The model under review builds one solid part; all positions refer to its coordinate system, in mm. A direction names the side the tool comes from. Round coordinates to 2 decimals unless told otherwise and drop trailing zeros. Loops run counter-clockwise (first coordinate to the right, second up) from the corner with the lowest first, then second, coordinate; pieces in that order, holes last. Notation, with made-up numbers: M -30,38 L -11,38 A24 ccw -11,65 Z; hole C 62.5,38.25 d4. An arc over 180 degrees is marked long. Answer in a Markdown table with one row per item. Add a question column.
from build123d import *

# Parameters (mm, degrees)
SKETCH2_W             = 31.8
SKETCH2_H             = 15.8
SKETCH2_W_2           = 29.4
SKETCH2_H_2           = 13.4
BOSS_EXTRUDE1_DEPTH   = 3.2
SKETCH2_3_R           = 3.255
SKETCH2_3_R_2         = 2.4
BOSS_EXTRUDE2_DEPTH   = 2.2
BOSS_EXTRUDE2_2_DEPTH = 2.2
BOSS_EXTRUDE2_3_DEPTH = 2.2
SKETCH3_W             = 29.4
SKETCH3_H             = 13.4
BOSS_EXTRUDE3_DEPTH   = 1
SKETCH4_R             = 2.4
SKETCH4_R_2           = 2.399999999
BOSS_EXTRUDE4_DEPTH   = 1.8
SKETCH5_R             = 1.3
CUT_EXTRUDE1_DEPTH    = 1.8


with BuildPart() as part:
    # Sketch2 → Boss-Extrude1 (new body)
    with BuildSketch(Plane.XY):
        with Locations((15.9, -7.9)):
            Rectangle(SKETCH2_W, SKETCH2_H)
        with Locations((15.9, -7.9)):
            Rectangle(SKETCH2_W_2, SKETCH2_H_2, mode=Mode.SUBTRACT)
    extrude(amount=-BOSS_EXTRUDE1_DEPTH)



with BuildPart() as body_2:
    # Sketch2<3> → Boss-Extrude2 (new body)
    with BuildSketch(Plane.XY):
        with Locations((23.9, -7.8)):
            Circle(SKETCH2_3_R)
        with Locations((23.9, -7.8)):
            Circle(SKETCH2_3_R_2, mode=Mode.SUBTRACT)
    extrude(amount=-BOSS_EXTRUDE2_DEPTH)


with BuildPart() as body_3:
    # Sketch2<3> → Boss-Extrude2 2 (new body)
    with BuildSketch(Plane.XY):
        with Locations((15.899999998, -7.8)):
            Circle(SKETCH2_3_R)
        with Locations((15.899999998, -7.8)):
            Circle(SKETCH2_3_R_2, mode=Mode.SUBTRACT)
    extrude(amount=-BOSS_EXTRUDE2_2_DEPTH)


with BuildPart() as body_4:
    # Sketch2<3> → Boss-Extrude2 3 (new body)
    with BuildSketch(Plane.XY):
        with Locations((7.899999996, -7.8)):
            Circle(SKETCH2_3_R)
        with Locations((7.899999996, -7.8)):
            Circle(SKETCH2_3_R_2, mode=Mode.SUBTRACT)
    extrude(amount=-BOSS_EXTRUDE2_3_DEPTH)


with BuildPart() as part_1:
    add(part.part)

    add(body_2.part)  # Boss-Extrude3 merges body 2

    add(body_3.part)  # Boss-Extrude3 merges body 3

    add(body_4.part)  # Boss-Extrude3 merges body 4
    # Sketch3 → Boss-Extrude3 (add)
    with BuildSketch(Plane(origin=(0, 0, -2.2), x_dir=(-1, 0, 0), z_dir=(0, 0, -1))):
        with Locations((-15.9, -7.9)):
            Rectangle(SKETCH3_W, SKETCH3_H)
    extrude(amount=BOSS_EXTRUDE3_DEPTH)

    # Sketch4 → Boss-Extrude4 (add)
    with BuildSketch(Plane(origin=(0, 0, -3.2), x_dir=(-1, 0, 0), z_dir=(0, 0, -1))):
        with Locations((-27.9, -3.9)):
            Circle(SKETCH4_R)
        with Locations((-19.899999998, -3.9)):
            Circle(SKETCH4_R)
        with Locations((-11.899999996, -3.9)):
            Circle(SKETCH4_R)
        with Locations((-3.899999994, -3.9)):
            Circle(SKETCH4_R)
        with Locations((-19.899999998, -11.9)):
            Circle(SKETCH4_R_2)
        with Locations((-11.899999996, -11.9)):
            Circle(SKETCH4_R_2)
        with Locations((-3.899999994, -11.9)):
            Circle(SKETCH4_R_2)
        with Locations((-27.9, -11.9)):
            Circle(SKETCH4_R_2)
    extrude(amount=BOSS_EXTRUDE4_DEPTH)

    # Sketch5 → Cut-Extrude1 (cut)
    with BuildSketch(Plane.XY.offset(-2.2)):
        with Locations((3.899999994, -3.9)):
            Circle(SKETCH5_R)
        with Locations((11.899999996, -3.9)):
            Circle(SKETCH5_R)
        with Locations((19.899999998, -3.9)):
            Circle(SKETCH5_R)
        with Locations((27.9, -3.9)):
            Circle(SKETCH5_R)
        with Locations((11.899999996, -11.900000002)):
            Circle(SKETCH5_R)
        with Locations((19.899999998, -11.900000002)):
            Circle(SKETCH5_R)
        with Locations((27.9, -11.900000002)):
            Circle(SKETCH5_R)
        with Locations((3.899999994, -11.900000002)):
            Circle(SKETCH5_R)
    extrude(amount=-CUT_EXTRUDE1_DEPTH, mode=Mode.SUBTRACT)


solid = part_1.part
1. Take a section at A-A, the plane z = -0.5. State the section outline as (x, y) points (3 decimals), and give its area (3 significant figures).
2. Take a section at D-D, the plane x = 15.9. State the section outline as (y, z) points (3 decimals), and give its area (3 significant figures).
3. For pin 1 Ø1.3 at (x, y) = (20.5, -4) entering from +Z; pin 2 Ø2.5 at (x, y) = (25, -8) entering from +Z; pin 3 Ø1.5 at (x, y) = (12, -8.5) entering from -Z, all flat-tipped, find the tip position at first contact; note any pin that passes through.
4. Mouldability with a two-part tool opening along Y and no side actions: class faces 1 (the flat face through (12, -12, -4)), 2 (the flat face through (20, -4, -4)), 3 (the flat face through (4, -12, -5)), 4 (the flat face through (16, 0, -2)) as released by +Y, released by -Y, zero draft, split by the parting line, or undercut.
5. Take a section at B-B, the plane x = 3.9. State the section outline as (y, z) points.
6. To check wall thickness, follow probe 1 along X at (y, z) = (-11.9, -2.7); probe 2 along Y at (x, z) = (7.9, -0.9) (3 decimals); probe 3 along Y at (x, z) = (19.9, -2.55). State the ranges of each line that lie inside material, in increasing order.
7. Machinability: for faces 5 (the flat face through (22, -10, 0)), 6 (the cylindrical face through (12.5, -13.053, -3.087)), 7 (the cylindrical face through (21.67, -10.28, -4.09)), which of the approach directions +Z, -Z, +X, -X, +Y, -Y give a long, thin tool a straight path to every point of the face, cutting with its end or side? Answer none if there is none.
Check sheet entries:
| question | item | result |
|---|---|---|
| 1 | outline | M 0,-15.8 L 31.8,-15.8 L 31.8,0 L 0,0 Z; C 7.9,-7.8 d6.51; C 15.9,-7.8 d6.51; C 23.9,-7.8 d6.51; hole M 1.2,-14.6 L 30.6,-14.6 L 30.6,-1.2 L 1.2,-1.2 Z; hole C 7.9,-7.8 d4.8; hole C 15.9,-7.8 d4.8; hole C 23.9,-7.8 d4.8 |
| 1 | area | 154 mm^2 |
| 2 | outline | M -15.8,-3.2 L 0,-3.2 L 0,0 L -1.2,0 L -1.2,-2.2 L -4.545,-2.2 L -4.545,0 L -5.4,0 L -5.4,-2.2 L -10.2,-2.2 L -10.2,0 L -11.055,0 L -11.055,-2.2 L -14.6,-2.2 L -14.6,0 L -15.8,0 Z |
| 2 | area | 24.8 mm^2 |
| 3 | pin 1 | stops at z = -4 |
| 3 | pin 2 | stops at z = -2.2 |
| 3 | pin 3 | stops at z = -3.2 |
| 4 | face 1 | undercut |
| 4 | face 2 | undercut |
| 4 | face 3 | zero draft |
| 4 | face 4 | released by +Y |
| 5 | outline | M -15.8,-3.2 L -14.3,-3.2 L -14.3,-5 L -9.5,-5 L -9.5,-3.2 L -6.3,-3.2 L -6.3,-5 L -1.5,-5 L -1.5,-3.2 L 0,-3.2 L 0,0 L -1.2,0 L -1.2,-2.2 L -2.6,-2.2 L -2.6,-4 L -5.2,-4 L -5.2,-2.2 L -10.6,-2.2 L -10.6,-4 L -13.2,-4 L -13.2,-2.2 L -14.6,-2.2 L -14.6,0 L -15.8,0 Z |
| 6 | probe 1 | x = 0 to 2.6, 5.2 to 10.6, 13.2 to 18.6, 21.2 to 26.6, 29.2 to 31.8 |
| 6 | probe 2 | y = -15.8 to -14.6, -11.055 to -10.2, -5.4 to -4.545, -1.2 to 0 |
| 6 | probe 3 | y = -15.8 to -13.2, -10.6 to -5.2, -2.6 to 0 |
| 7 | face 5 | +Z, +X, -X, +Y, -Y |
| 7 | face 6 | +Z |
| 7 | face 7 | -Z |
